from build123d import *

# Parameters (mm, degrees)
F0_R     = 3.81
F1_DEPTH = 35.306
F2_R     = 6.35
F3_DEPTH = 12.7
F4_R     = 8.89
F5_DEPTH = 9.652
F6_R     = 10.16
F7_DEPTH = 6.35
F8_R     = 11.43
F9_DEPTH = 3.048


# Not quite as in the source:
# - the program builds the solid bodies; features that only make, move or delete a surface that nothing else refers to are left out


with BuildPart() as f1:
    # F0 (on Front) → F1 (new body)
    with BuildSketch(Plane.XZ):
        Circle(F0_R)
    extrude(amount=F1_DEPTH)

    # F2 (on Front) → F3 (join)
    with BuildSketch(Plane.XZ):
        Circle(F2_R)
    extrude(amount=F3_DEPTH)

    # F4 (on Front) → F5 (join)
    with BuildSketch(Plane.XZ):
        Circle(F4_R)
    extrude(amount=F5_DEPTH)

    # F6 (on Front) → F7 (join)
    with BuildSketch(Plane.XZ):
        Circle(F6_R)
    extrude(amount=F7_DEPTH)

    # F8 (on Front) → F9 (join)
    with BuildSketch(Plane.XZ):
        Circle(F8_R)
    extrude(amount=F9_DEPTH)


solid = f1.part
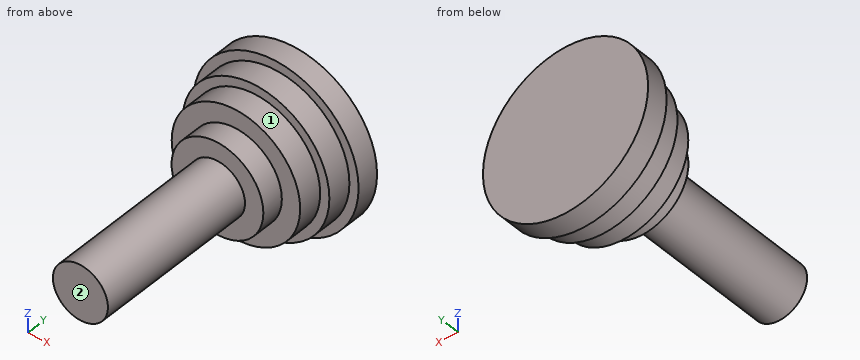
The model under review builds one solid part; all positions refer to its coordinate system, in mm. Face numbers are marked on the shaded views. A direction names the side the tool comes from. Give positions to 0.01 mm unless a question says otherwise; leave off trailing zeros. Write each loop counter-clockwise with the first axis right and the second up, starting at its lowest first coordinate (ties: lowest second). Pieces come first, ordered by that corner, then holes.
1. Tool access review of the marked faces 1 and 2: name each direction out of +Z, -Z, +X, -X, +Y, -Y from which nothing blocks a thin tool from reaching the whole face with its end or side.
2. Wall thickness on L1, parallel to Y at x = -4.5, z = 5.75; L2, parallel to Y at x = -8.25, z = 6.25; L3, parallel to X at y = -7.5, z = 4.75: over which ranges is each line inside the solid? List them lowest first.
3. Add section B-B, the plane z = 0. Write out the cut boundary in (x, y), plus the area to 3 significant figures.
4. Add section D-D, the plane x = 0. Write out the cut boundary in (y, z).
5. Add section C-C, the plane y = -21. Write out the cut boundary in (x, z), plus the area to 3 significant figures.
6. Add section A-A, the plane x = -5. Write out the cut boundary in (y, z), plus the area to 3 significant figures.
7. For P1, Ø1, axis at y = -6, z = 2, coming from the -X side; P2, Ø2, axis at x = 2, y = -10.5, coming from the -Z side; P3, Ø2, axis at x = -4.5, z = -5, coming from the +Y side; P4, Ø1.5, axis at y = -13.5, z = 7.5, coming from the +X side, all flat-tipped, find the tip position at first contact; note any pin that passes through.
Worked answers:
1. face 1: -Y
1. face 2: +Z, -Z, +X, -X, -Y
2. L1: y = -9.65 to 0
2. L2: y = -3.05 to 0
2. L3: x = -7.51 to 7.51
3. outline: (-11.43, -3.05) - (-10.16, -3.05) - (-10.16, -6.35) - (-8.89, -6.35) - (-8.89, -9.65) - (-6.35, -9.65) - (-6.35, -12.7) - (-3.81, -12.7) - (-3.81, -35.31) - (3.81, -35.31) - (3.81, -12.7) - (6.35, -12.7) - (6.35, -9.65) - (8.89, -9.65) - (8.89, -6.35) - (10.16, -6.35) - (10.16, -3.05) - (11.43, -3.05) - (11.43, 0) - (-11.43, 0) - close
3. area: 406 mm2
4. outline: (-35.31, -3.81) - (-12.7, -3.81) - (-12.7, -6.35) - (-9.65, -6.35) - (-9.65, -8.89) - (-6.35, -8.89) - (-6.35, -10.16) - (-3.05, -10.16) - (-3.05, -11.43) - (0, -11.43) - (0, 11.43) - (-3.05, 11.43) - (-3.05, 10.16) - (-6.35, 10.16) - (-6.35, 8.89) - (-9.65, 8.89) - (-9.65, 6.35) - (-12.7, 6.35) - (-12.7, 3.81) - (-35.31, 3.81) - close
5. outline: circle Ø7.62 at (0, 0)
5. area: 45.6 mm2
6. outline: (-12.7, -3.91) - (-9.65, -3.91) - (-9.65, -7.35) - (-6.35, -7.35) - (-6.35, -8.84) - (-3.05, -8.84) - (-3.05, -10.28) - (0, -10.28) - (0, 10.28) - (-3.05, 10.28) - (-3.05, 8.84) - (-6.35, 8.84) - (-6.35, 7.35) - (-9.65, 7.35) - (-9.65, 3.91) - (-12.7, 3.91) - close
6. area: 193 mm2
7. P1: stops at x = -10.05
7. P2: stops at z = -8.77
7. P3: stops at y = 0
7. P4: passes through
